```python
from build123d import *

# Parameters (mm, degrees)
SKETCH_1_W          = 60
SKETCH_1_H          = 50
EXTRUDE_1_DEPTH     = 6
SKETCH_2_W          = 60
SKETCH_2_H          = 10
EXTRUDE_3_DEPTH     = 30
SKETCH_3_W          = 60
SKETCH_3_H          = 5
EXTRUDE_4_DEPTH     = 4
SKETCH_4_W          = 60
SKETCH_4_H          = 5
EXTRUDE_5_DEPTH     = 4
SKETCH_6_R          = 1.555741847
SKETCH_6_R_2        = 1.533074906
SKETCH_6_R_3        = 1.574012297
CUT_EXTRUDE_1_DEPTH = 60.093146811
SKETCH_7_R          = 1.55
CUT_EXTRUDE_2_DEPTH = 60.093146811
SKETCH_9_W          = 60
SKETCH_9_H          = 28
SKETCH_9_W_2        = 40.4
SKETCH_9_H_2        = 20.5
EXTRUDE_6_DEPTH     = 28.1
SKETCH_11_R         = 5
CUT_EXTRUDE_3_DEPTH = 10
SKETCH_12_R         = 2.25
CUT_EXTRUDE_4_DEPTH = 16
CUT_EXTRUDE_5_DEPTH = 61.967204299


with BuildPart() as part:
    # 草图1 → 凸台-拉伸1 (new body)
    with BuildSketch(Plane.XY):
        Rectangle(SKETCH_1_W, SKETCH_1_H)
    extrude(amount=EXTRUDE_1_DEPTH)

    # 草图2 → 凸台-拉伸3 (add)
    with BuildSketch(Plane.XY.offset(6)):
        with Locations((0, 20)):
            Rectangle(SKETCH_2_W, SKETCH_2_H)
        with Locations((0, -20)):
            Rectangle(SKETCH_2_W, SKETCH_2_H)
    extrude(amount=EXTRUDE_3_DEPTH)

    # 草图3 → 凸台-拉伸4 (add)
    with BuildSketch(Plane(origin=(0, -15, 0), x_dir=(1, 0, 0), z_dir=(0, 1, 0))):
        with Locations((0, -33.5)):
            Rectangle(SKETCH_3_W, SKETCH_3_H)
    extrude(amount=EXTRUDE_4_DEPTH)

    # 草图4 → 凸台-拉伸5 (add)
    with BuildSketch(Plane.XZ.offset(-15)):
        with Locations((0, 33.5)):
            Rectangle(SKETCH_4_W, SKETCH_4_H)
    extrude(amount=EXTRUDE_5_DEPTH)

    # 草图6 → 切除-拉伸1 (cut, through all)
    with BuildSketch(Plane(origin=(0, -11, 0), x_dir=(1, 0, 0), z_dir=(0, 1, 0))):
        with Locations(Location((-13.5, -33.5, 0), (0, 0, 270))):
            Circle(SKETCH_6_R)
        with Locations(Location((1.5, -33.5, 0), (0, 0, 270))):
            Circle(SKETCH_6_R_2)
        with Locations(Location((16.5, -33.5, 0), (0, 0, 270))):
            Circle(SKETCH_6_R_3)
    extrude(amount=-CUT_EXTRUDE_1_DEPTH, mode=Mode.SUBTRACT)

    # 草图7 → 切除-拉伸2 (cut, through all)
    with BuildSketch(Plane.XZ.offset(-11)):
        with Locations(Location((16.5, 33.5, 0), (0, 0, 270))):
            Circle(SKETCH_7_R)
        with Locations(Location((1.5, 33.5, 0), (0, 0, 270))):
            Circle(SKETCH_7_R)
        with Locations(Location((-13.5, 33.5, 0), (0, 0, 270))):
            Circle(SKETCH_7_R)
    extrude(amount=-CUT_EXTRUDE_2_DEPTH, mode=Mode.SUBTRACT)

    # 草图9 → 凸台-拉伸6 (add)
    with BuildSketch(Plane(origin=(0, 0, 0), x_dir=(-1, 0, 0), z_dir=(0, 0, -1))):
        Rectangle(SKETCH_9_W, SKETCH_9_H)
        Rectangle(SKETCH_9_W_2, SKETCH_9_H_2, mode=Mode.SUBTRACT)
    extrude(amount=EXTRUDE_6_DEPTH)

    # 草图11 → 切除-拉伸3 (cut)
    with BuildSketch(Plane(origin=(30, 0, 0), x_dir=(0, 0, -1), z_dir=(1, 0, 0))):
        with Locations((5.781700187, 0)):
            Circle(SKETCH_11_R)
    extrude(amount=-CUT_EXTRUDE_3_DEPTH, mode=Mode.SUBTRACT)

    # 草图12 → 切除-拉伸4 (cut)
    with BuildSketch(Plane(origin=(0, 0, -28.1), x_dir=(-1, 0, 0), z_dir=(0, 0, -1))):
        with Locations((24.8, -5)):
            Circle(SKETCH_12_R)
        with Locations((24.8, 5)):
            Circle(SKETCH_12_R)
        with Locations((-24.8, -5)):
            Circle(SKETCH_12_R)
        with Locations((-24.8, 5)):
            Circle(SKETCH_12_R)
    extrude(amount=-CUT_EXTRUDE_4_DEPTH, mode=Mode.SUBTRACT)

    # 草图13 → 切除-拉伸5 (cut, through all)
    with BuildSketch(Plane(origin=(0, 14, 0), x_dir=(1, 0, 0), z_dir=(0, 1, 0))):
        Polygon((-12, 14.518770095), (-6, 4.12646525), (6, 4.12646525), (12, 14.518770095), (6, 24.911074941), (-6, 24.911074941), align=None)
    extrude(amount=-CUT_EXTRUDE_5_DEPTH, mode=Mode.SUBTRACT)


solid = part.part
```
Check sheet for the modelled part. Datum: model origin and axes. Units: mm. A direction names the side the tool comes from. Coordinates: 2 decimals unless noted, no trailing zeros. Write each loop counter-clockwise with the first axis right and the second up, starting at its lowest first coordinate (ties: lowest second). Pieces come first, ordered by that corner, then holes. Notation, with made-up numbers: M -15.5,70 L 23.5,70 A36 cw 23.5,105 Z; hole C 85.25,47.25 d11. An arc over 180 degrees is marked long. Write item = value, one per line. Start each with the question number.
1. Thickness scan on probe 1 along X at (y, z) = (-20.5, 33.5); probe 2 along Y at (x, z) = (22, 23); probe 3 along X at (y, z) = (7, -2). Record the ranges inside material, lowest first.
2. Sectioned sample at D-D (z = -13). Record the cut outline in (x, y), then the cut area to 3 significant figures.
3. Mould release check, pull along Y, two halves, no side actions. Record for faces 4 (the flat face through (0, -25, 18)), 5 (the flat face through (0, -12, -4.126)), 6 (the cylindrical face through (-22.552, 5.099, -20.212)), 7 (the flat face through (0, -13, 31)): pulls with the +Y half, pulls with the -Y half, needs draft (parallel to the pull), parting line crosses it, or undercut.
4. Sectioned sample at B-B (x = 16.5). Record the cut outline in (y, z).
5. Sectioned sample at C-C (z = 18.5). Record the cut outline in (x, y).
6. Tool access check on faces 1 (the flat face through (9, -10.25, -8)), 2 (the flat face through (0, 20, 0)), 3 (the flat face through (-8.958, 12.151, -19.788)). Record the directions out of +Z, -Z, +X, -X, +Y, -Y that give a thin tool (end or side, any length) a straight path to the whole face; none if there is none.
7. Go/stop test with flat-tipped pins: pin 1 (1 mm diameter, centred on x = -22, y = 17, fed in from -Z); pin 2 (3 mm diameter, centred on x = 9.5, z = -7, fed in from +Y); pin 3 (12 mm diameter, centred on x = 9.5, z = -19.5, fed in from -Y). Record where each tip stops, or that it passes through.
8. Sectioned sample at A-A (z = 33.5). State how many separate pieces and enclosed holes the cut face has, then the cut area to 3 significant figures.
The answers:
q1.probe_1 = -30 to -15.06, -11.94 to -0.03, 3.03 to 14.93, 18.07 to 30
q1.probe_2 = -25 to -15, 15 to 25
q1.probe_3 = -30 to -20.2, 20.2 to 30
q2.outline = M -30,-14 L -11.12,-14 L -11.12,-10.25 L -20.2,-10.25 L -20.2,10.25 L -11.12,10.25 L -11.12,14 L -30,14 Z; M 11.12,-14 L 30,-14 L 30,14 L 11.12,14 L 11.12,10.25 L 20.2,10.25 L 20.2,-10.25 L 11.12,-10.25 Z; hole C -24.8,-5 d4.5; hole C -24.8,5 d4.5; hole C 24.8,-5 d4.5; hole C 24.8,5 d4.5
q2.area = 621 mm²
q3.face_4 = pulls with the -Y half
q3.face_5 = needs draft
q3.face_6 = undercut
q3.face_7 = undercut
q4.outline = M -25,0 L -14,0 L -14,-28.1 L -10.25,-28.1 L -10.25,0 L 10.25,0 L 10.25,-28.1 L 14,-28.1 L 14,0 L 25,0 L 25,31.95 L 11,31.95 L 11,31 L 15,31 L 15,6 L -15,6 L -15,31 L -11,31 L -11,31.93 L -25,31.93 Z; M -25,35.07 L -11,35.07 L -11,36 L -25,36 Z; M 11,35.05 L 25,35.05 L 25,36 L 11,36 Z
q5.outline = M -30,-25 L 30,-25 L 30,-15 L -30,-15 Z; M -30,15 L 30,15 L 30,25 L -30,25 Z
q6.face_1 = -Z
q6.face_2 = -Z, +X, -X, +Y
q6.face_3 = +Y, -Y
q7.pin_1 = 0
q7.pin_2 = 14
q7.pin_3 = -14
q8.separate_pieces = 8
q8.enclosed_holes = 0
q8.area = 1,420 mm²
